Input: part model. Units: mm. Frame: model coordinates. A direction names the side the tool comes from. Coordinates: 2 decimals unless noted, no trailing zeros. Loops run counter-clockwise (first coordinate to the right, second up) from the corner with the lowest first, then second, coordinate; pieces in that order, holes last.
(1) Contact query for flat-ended pins moving along their axis: P1, Ø16.5, axis at y = 24.5, z = 3, coming from the +X side; P2, Ø16.5, axis at y = 19.5, z = -9, coming from the -X side; P3, Ø8, axis at y = 6, z = 0, coming from the -X side; P4, Ø3, axis at x = 27.49, z = -8.25, coming from the -Y side. Output: stop coordinate, or through.
(2) Section B-B, the plane x = 23. Return loops of the section in (y, z), then the cut area to 3 significant figures.
(3) Mould query, pull axis Z, two halves, no side actions, for faces 4 (the face through (13, 27.2, 0)), 5 (the face through (33.25, 30.14, 0.24)), 6 (the face through (11.91, 32.11, 15.32)). Classes: released by +Z, released by -Z, zero draft, split by the parting line, or undercut.
(4) Line query: L1, parallel to X at y = 20.5, z = 4; L2, parallel to Y at x = 24, z = 15; L3, parallel to X at y = 32.6, z = -8.25. Output: solid intervals per line, ascending.
(5) Section A-A, the plane y = 17. Return loops of the section in (x, z), then the cut area to 3 significant figures.
(6) Section D-D, the plane y = 6. Give the number of separate pieces and of enclosed holes in the cut face, then the cut area to 3 significant figures.
(7) Set-up query: faces 1 (the face through (4, 14, 0)), 2 (the face through (29, 31.2, -10)), 3 (the face through (-3, 27.2, 3)). Return all of +Z, -Z, +X, -X, +Y, -Y with unobstructed straight access to the full face (end or side cutting, diameter ignored); none if empty.
(8) Section C-C, the plane z = 2. Return loops of the section in (x, y), then the cut area to 3 significant figures.
```python
from build123d import *

# Parameters (mm, degrees)
EXTRUDE_1_DEPTH     = 24
SKETCH_3_R          = 3.15
CUT_EXTRUDE_2_DEPTH = 26.4
SKETCH_4_R          = 20.05
EXTRUDE_2_DEPTH     = 5.8
SKETCH_5_R          = 1.75
CUT_EXTRUDE_3_DEPTH = 5.8
SKETCH_6_R          = 3.1
CUT_EXTRUDE_4_DEPTH = 4
SKETCH_6_3_R        = 3.1
CUT_EXTRUDE_5_DEPTH = 6


with BuildPart() as part:
    # 草圖1 → 填料-伸長1 (new body, symmetric)
    with BuildSketch(Plane.XY):
        Polygon((0, 0), (0, 33), (26.4, 33), (26.4, 0), (22.4, 0), (22.4, 27.2), (4, 27.2), (4, 0), align=None)
    extrude(amount=EXTRUDE_1_DEPTH, both=True)

    # 草圖3 → 除料-伸長2 (cut)
    with BuildSketch(Plane(origin=(26.4, 0, 0), x_dir=(0, 0, -1), z_dir=(1, 0, 0))):
        with Locations((0, 6)):
            Circle(SKETCH_3_R)
        with Locations((15, 6)):
            Circle(SKETCH_3_R)
        with Locations((-15, 6)):
            Circle(SKETCH_3_R)
    extrude(amount=-CUT_EXTRUDE_2_DEPTH, mode=Mode.SUBTRACT)

    # 草圖4 → 填料-伸長2 (add)
    with BuildSketch(Plane(origin=(0, 33, 0), x_dir=(1, 0, 0), z_dir=(0, 1, 0))):
        with Locations((13.2, 0)):
            Circle(SKETCH_4_R)
    extrude(amount=-EXTRUDE_2_DEPTH)

    # 草圖5 → 除料-伸長3 (cut)
    with BuildSketch(Plane(origin=(0, 33, 0), x_dir=(1, 0, 0), z_dir=(0, 1, 0))):
        with Locations((13.2, -16.5)):
            Circle(SKETCH_5_R)
        with Locations((-1.089419162, 8.25)):
            Circle(SKETCH_5_R)
        with Locations((27.489419162, 8.25)):
            Circle(SKETCH_5_R)
    extrude(amount=-CUT_EXTRUDE_3_DEPTH, mode=Mode.SUBTRACT)

    # 草圖6 → 除料-伸長4 (cut)
    with BuildSketch(Plane.XZ.offset(-27.2)):
        with Locations((-1.089419162, -8.25)):
            Circle(SKETCH_6_R)
        with Locations((13.2, 16.5)):
            Circle(SKETCH_6_R)
        with Locations((27.489419162, -8.25)):
            Circle(SKETCH_6_R)
    extrude(amount=-CUT_EXTRUDE_4_DEPTH, mode=Mode.SUBTRACT)

    # 草圖6<3> → 除料-伸長5 (cut)
    with BuildSketch(Plane.XZ.offset(-27.2)):
        with Locations((-1.089419162, -8.25)):
            Circle(SKETCH_6_3_R)
        with Locations((27.489419162, -8.25)):
            Circle(SKETCH_6_3_R)
    extrude(amount=CUT_EXTRUDE_5_DEPTH, mode=Mode.SUBTRACT)


solid = part.part
```
Report:
1. P1: stops at x = 33.25
1. P2: stops at x = -5.92
1. P3: stops at x = 0
1. P4: stops at y = 0
2. outline: (0, -24) - (33, -24) - (33, 24) - (0, 24) - close; hole circle Ø6.3 at (6, -15); hole circle Ø6.3 at (6, 0); hole circle Ø6.3 at (6, 15)
2. area: 1,490 mm2
3. face 4: zero draft
3. face 5: split by the parting line
3. face 6: undercut
4. L1: x = 0 to 4, 22.4 to 26.4
4. L2: y = 0 to 2.85, 9.15 to 33
4. L3: x = -5.07 to -2.84, 0.66 to 25.74, 29.24 to 31.47
5. outline: (0, -24) - (4, -24) - (4, 24) - (0, 24) - close; (22.4, -24) - (26.4, -24) - (26.4, 24) - (22.4, 24) - close
5. area: 384 mm2
6. separate pieces: 8
6. enclosed holes: 0
6. area: 233 mm2
7. face 1: +Z, -Z, -Y
7. face 2: none
7. face 3: +Z, -Z, -X, -Y
8. outline: (-6.75, 27.2) - (0, 27.2) - (0, 8.43) - (4, 8.43) - (4, 27.2) - (22.4, 27.2) - (22.4, 8.43) - (26.4, 8.43) - (26.4, 27.2) - (33.15, 27.2) - (33.15, 33) - (-6.75, 33) - close; (0, 0) - (4, 0) - (4, 3.57) - (0, 3.57) - close; (22.4, 0) - (26.4, 0) - (26.4, 3.57) - (22.4, 3.57) - close
8. area: 410 mm2
